The listing builds one solid part. Answer for the finished solid, in the listing's coordinates (mm). Face numbers are marked on the shaded views. Coordinates: 2 decimals unless noted, no trailing zeros. Loops run counter-clockwise (first coordinate to the right, second up) from the corner with the lowest first, then second, coordinate; pieces in that order, holes last. Notation, with made-up numbers: (62.5, 1.5) - (94.5, 1.5) arc R22 ccw to (94.5, 38.5) - close; hole circle Ø6 at (64, 56.5). An arc over 180 degrees is marked (long way). One line per question, with ' | ' between items.
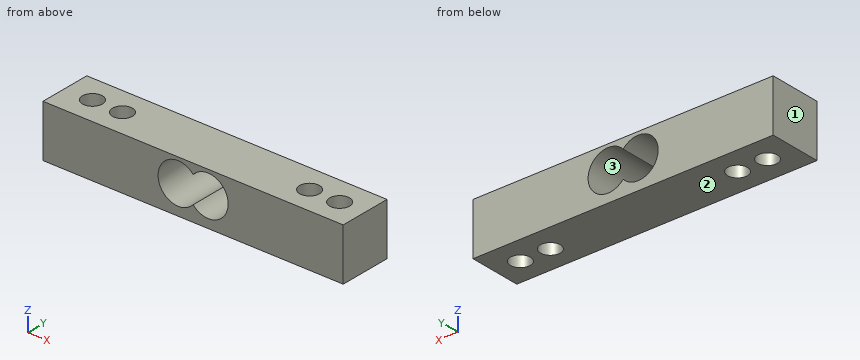
from build123d import *

# Parameters (mm, degrees)
SKETCH1_W           = 75
SKETCH1_H           = 13
BOSS_EXTRUDE1_DEPTH = 13
SKETCH3_R           = 2.5
CUT_EXTRUDE4_DEPTH  = 13
CUT_EXTRUDE5_DEPTH  = 13


with BuildPart() as part:
    # Sketch1 → Boss-Extrude1 (new body)
    with BuildSketch(Plane.XY):
        Rectangle(SKETCH1_W, SKETCH1_H)
    extrude(amount=BOSS_EXTRUDE1_DEPTH)

    # Sketch3 → Cut-Extrude4 (cut)
    with BuildSketch(Plane.XY):
        with Locations(Location((31.216304174, -0.096660898, 0), (0, 0, 180))):
            Circle(SKETCH3_R)
        with Locations(Location((23.716304174, -0.096660898, 0), (0, 0, 180))):
            Circle(SKETCH3_R)
        with Locations(Location((-23.119138504, 0.000687163, 0), (0, 0, 180))):
            Circle(SKETCH3_R)
        with Locations(Location((-30.619138504, 0.000687163, 0), (0, 0, 180))):
            Circle(SKETCH3_R)
    extrude(amount=CUT_EXTRUDE4_DEPTH, mode=Mode.SUBTRACT)

    # Sketch4 → Cut-Extrude5 (cut)
    with BuildSketch(Plane(origin=(0, 6.5, 0), x_dir=(1, 0, 0), z_dir=(0, 1, 0))):
        with BuildLine():
            ThreePointArc((0, -3.877187484), (-8.75, -7.184376623), (0, -10.491565762))
            ThreePointArc((0, -10.491565762), (8.75, -7.184376623), (0, -3.877187484))
        make_face()
    extrude(amount=-CUT_EXTRUDE5_DEPTH, mode=Mode.SUBTRACT)


solid = part.part
Item 1: Find section D-D, the plane z = 11.25. Write down the section's boundary in (x, y), plus the area to 3 significant figures.
Taken from the geometry:
outline: (-37.5, -6.5) - (-6.66, -6.5) - (-6.66, 6.5) - (-37.5, 6.5) - close; (-0.84, -6.5) - (0.84, -6.5) - (0.84, 6.5) - (-0.84, 6.5) - close; (6.66, -6.5) - (37.5, -6.5) - (37.5, 6.5) - (6.66, 6.5) - close; hole circle Ø5 at (-30.62, 0); hole circle Ø5 at (-23.12, 0); hole circle Ø5 at (23.72, -0.1); hole circle Ø5 at (31.22, -0.1) | area: 745 mm2
Item 2: This flat-tipped pin is pushed along its axis until it touches: pin 1 Ø3 at (x, y) = (31.22, -0.1) entering from -Z. Where does it stop, or does it pass through?
Taken from the geometry:
pin 1: passes through
Item 3: Find section C-C, the plane z = 6.75. Write down the section's boundary in (x, y), plus the area to 3 significant figures.
Taken from the geometry:
outline: (-37.5, -6.5) - (-8.73, -6.5) - (-8.73, 6.5) - (-37.5, 6.5) - close; (8.73, -6.5) - (37.5, -6.5) - (37.5, 6.5) - (8.73, 6.5) - close; hole circle Ø5 at (-30.62, 0); hole circle Ø5 at (-23.12, 0); hole circle Ø5 at (23.72, -0.1); hole circle Ø5 at (31.22, -0.1) | area: 669 mm2
Item 4: Find the intervals of material crossed by line 1 (Z direction, x = -3.75, y = 1.5); line 2 (X direction, y = 0.75, z = 4.5); line 3 (X direction, y = -2, z = 8.5), in increasing order. Write a range as [from, to].
Taken from the geometry:
line 1: z = [0, 2.18], [12.18, 13] | line 2: x = [-37.5, -33], [-28.23, -25.5], [-20.73, -7.97], [7.97, 21.36], [26.07, 28.86], [33.57, 37.5] | line 3: x = [-37.5, -32.12], [-29.12, -24.62], [-21.62, -8.57], [8.57, 22.1], [25.34, 29.6], [32.84, 37.5]
Item 5: Find section B-B, the plane y = 1. Write down the section's boundary in (x, z).
Taken from the geometry:
outline: (-37.5, 0) - (-32.91, 0) - (-32.91, 13) - (-37.5, 13) - close; (-28.33, 0) - (-25.41, 0) - (-25.41, 13) - (-28.33, 13) - close; (-20.83, 0) - (21.47, 0) - (21.47, 13) - (-20.83, 13) - close; (25.96, 0) - (28.97, 0) - (28.97, 13) - (25.96, 13) - close; (33.46, 0) - (37.5, 0) - (37.5, 13) - (33.46, 13) - close; hole (0, 3.88) arc R5 ccw (long way) to (0, 10.49) arc R5 ccw (long way) to start
Item 6: Find section A-A, the plane x = -3.75. Write down the section's boundary in (y, z), plus the area to 3 significant figures.
Taken from the geometry:
outline: (-6.5, 0) - (6.5, 0) - (6.5, 2.18) - (-6.5, 2.18) - close; (-6.5, 12.18) - (6.5, 12.18) - (6.5, 13) - (-6.5, 13) - close | area: 39.0 mm2
Item 7: The mould has two halves that part along Z. Classify the marked faces 1, 2 and 3: pulls with the +Z half, pulls with the -Z half, needs draft (parallel to the pull), parting line crosses it, or undercut.
Taken from the geometry:
face 1: needs draft | face 2: pulls with the -Z half | face 3: undercut
